The listing builds one solid part. Answer for the finished solid, in the listing's coordinates (mm). Give positions to 0.01 mm unless a question says otherwise; leave off trailing zeros. Write each loop counter-clockwise with the first axis right and the second up, starting at its lowest first coordinate (ties: lowest second). Pieces come first, ordered by that corner, then holes. Notation, with made-up numbers: M 62.25,-26 L 81.25,-26 A5 ccw 81.25,-19 Z; hole C 72,27 d8. An arc over 180 degrees is marked long. Return JSON: item names as keys, results as strings.
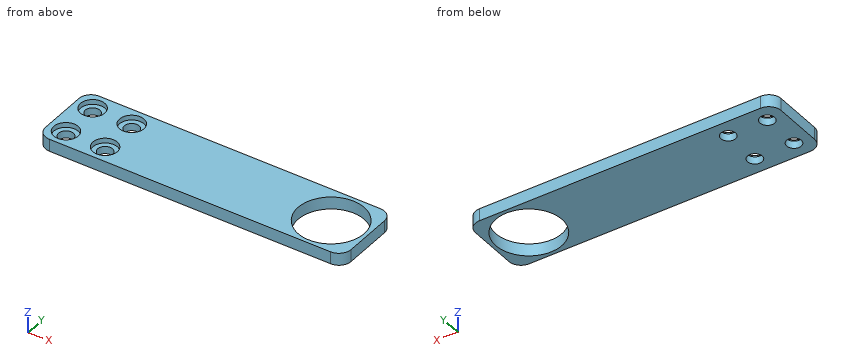
Autodesk Fusion 360 part; units mm, degrees
sketch "Sketch1" plane through (0, 0, 0) normal (0, 0, 1) x (1, 0, 0)
  line L0 (0, 0) -> (125, 0)
  line L1 (125, 0) -> (125, 30)
  line L2 (125, 30) -> (0, 30)
  line L3 (0, 30) -> (0, 0)
  dimension "d1" = 125
  dimension "d2" = 30
extrude "Extrude1" add sketch "Sketch1" along normal blind 5
sketch "Sketch2" plane through (0, 0, 5) normal (0, 0, 1) x (-1, 0, 0)
  line L0 (0, -30) -> (0, 0)
  line L1 (0, 0) -> (-125, 0)
  line L2 (-125, 0) -> (-125, -30)
  line L3 (-125, -30) -> (0, -30)
  circle A0 centre (-110, -15) radius 13.5
  dimension "d5" = 27
extrude "Extrude2" cut sketch "Sketch2" against normal blind 5 contours A0
sketch "Sketch3" plane through (0, 0, 5) normal (0, 0, 1) x (-1, 0, 0)
  circle A0 centre (-110, -15) radius 13.5
  line L0 (0, -30) -> (0, 0)
  line L1 (0, 0) -> (-125, 0)
  line L2 (-125, 0) -> (-125, -30)
  line L3 (-125, -30) -> (0, -30)
  circle A1 centre (-7, -23) radius 3
  circle A2 centre (-7, -7) radius 3
  circle A3 centre (-23, -23) radius 3
  circle A4 centre (-23, -7) radius 3
  dimension "d8" = 6
  dimension "d9" = 6
  dimension "d10" = 6
  dimension "d11" = 6
extrude "Extrude3" cut sketch "Sketch3" against normal blind 5 contours A1 | A2 | A3 | A4
sketch "Sketch4" plane through (0, 0, 5) normal (0, 0, 1) x (-1, 0, 0)
  circle A0 centre (-23, -7) radius 3
  circle A1 centre (-23, -23) radius 3
  circle A2 centre (-7, -7) radius 3
  circle A3 centre (-7, -23) radius 3
  circle A4 centre (-110, -15) radius 13.5
  line L0 (0, -30) -> (0, 0)
  line L1 (0, 0) -> (-125, 0)
  line L2 (-125, 0) -> (-125, -30)
  line L3 (-125, -30) -> (0, -30)
  circle A5 centre (-7, -23) radius 5
  circle A6 centre (-23, -23) radius 5
  circle A7 centre (-7, -7) radius 5
  circle A8 centre (-23, -7) radius 5
  dimension "d14" = 10
  dimension "d15" = 10
  dimension "d16" = 10
  dimension "d17" = 10
extrude "Extrude4" cut sketch "Sketch4" against normal blind 2 contours A5 | A6 | A7 | A8
fillet "Fillet1" radius 5 4 edges at (125, 30, 2.5) (125, 0, 2.5) (0, 0, 2.5) (0, 30, 2.5)
Item 1: A cutting plane is placed at B-B, the plane z = 1. Write down the section's boundary in (x, y).
Geometry results:
{"outline": "M 0,5 A5 ccw 5,0 L 120,0 A5 ccw 125,5 L 125,25 A5 ccw 120,30 L 5,30 A5 ccw 0,25 Z; hole C 7,7 d6; hole C 7,23 d6; hole C 23,7 d6; hole C 23,23 d6; hole C 110,15 d27"}
Item 2: Given pin 1 Ø9.5 at (x, y) = (7, 7) entering from +Z, flat-ended and moving along its own axis, determine where the tip first touches the part or whether it passes through.
Geometry results:
{"pin 1": "stops at z = 3"}
Item 3: A cutting plane is placed at C-C, the plane x = 110. Write down the section's boundary in (y, z).
Geometry results:
{"outline": "M 0,0 L 1.5,0 L 1.5,5 L 0,5 Z; M 28.5,0 L 30,0 L 30,5 L 28.5,5 Z"}
Item 4: A cutting plane is placed at A-A, the plane x = 7. Write down the section's boundary in (y, z), plus the area to 3 significant figures.
Geometry results:
{"outline": "M 0,0 L 4,0 L 4,3 L 2,3 L 2,5 L 0,5 Z; M 10,0 L 20,0 L 20,3 L 18,3 L 18,5 L 12,5 L 12,3 L 10,3 Z; M 26,0 L 30,0 L 30,5 L 28,5 L 28,3 L 26,3 Z", "area": "74.0 mm2"}
Item 5: A cutting plane is placed at D-D, the plane y = 21.5. Write down the section's boundary in (x, z).
Geometry results:
{"outline": "M 0,0 L 4.4,0 L 4.4,3 L 2.23,3 L 2.23,5 L 0,5 Z; M 9.6,0 L 20.4,0 L 20.4,3 L 18.23,3 L 18.23,5 L 11.77,5 L 11.77,3 L 9.6,3 Z; M 25.6,0 L 98.17,0 L 98.17,5 L 27.77,5 L 27.77,3 L 25.6,3 Z; M 121.83,0 L 125,0 L 125,5 L 121.83,5 Z"}
Item 6: Find the intervals of material crossed by line 1 (Y direction, x = 23, z = 4.1); line 2 (Y direction, x = 7, z = 1.25); line 3 (X direction, y = 23, z = 1.6), in increasing order.
Geometry results:
{"line 1": "y = 0 to 2, 12 to 18, 28 to 30", "line 2": "y = 0 to 4, 10 to 20, 26 to 30", "line 3": "x = 0 to 4, 10 to 20, 26 to 99.13, 120.87 to 125"}
